For this review, take the finished solid that the model builds, in its own axes (mm). Face numbers are marked on the shaded views. Round coordinates to 2 decimals unless told otherwise and drop trailing zeros. Write each loop counter-clockwise with the first axis right and the second up, starting at its lowest first coordinate (ties: lowest second). Pieces come first, ordered by that corner, then holes. Notation, with made-up numbers: M -40,9.5 L -27,9.5 A13 cw -27,27.5 Z; hole C 45.5,79 d1. An arc over 180 degrees is marked long. Use one line per item in the form item = value. Start each with the question number.
Item 1: For P1, Ø1, axis at x = 5, y = 0.5, coming from the +Z side; P2, Ø2, axis at x = 25.5, y = 1, coming from the -Z side; P3, Ø3, axis at x = -30, z = 10, coming from the -Y side; P4, Ø0.6, axis at x = -25.5, y = 1, coming from the -Z side, all flat-tipped, find the tip position at first contact; note any pin that passes through.
Item 2: Draft analysis for pull direction X (two halves, no side actions). For the marked faces 1 and 2, state which applies: released by +X, released by -X, zero draft, split by the parting line, or undercut.
Item 3: Add section B-B (x = 30). Count the separate pieces of the cut face and the enclosed holes in it, and give its area (3 significant figures).
Item 4: For line 1 (X direction, y = 1.95, z = 10); line 2 (Z direction, x = 30, y = 1.8); line 3 (X direction, y = 1.7, z = 20), list the stretches that pass through material, from the lowest coordinate up. Write a range as [from, to].
Item 5: Add section A-A (y = 2.9). State the section outline as (x, z) points.
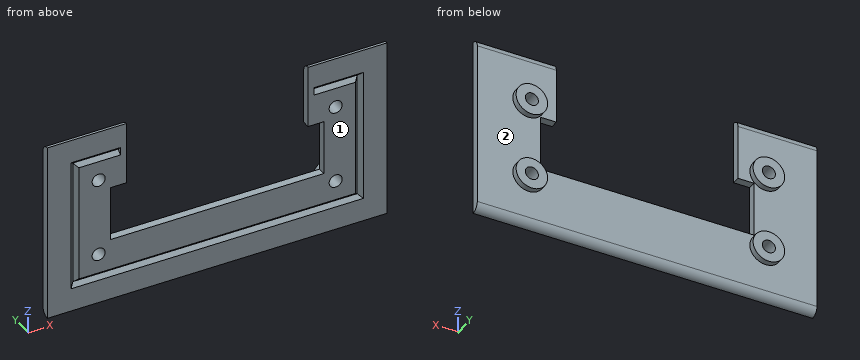
from build123d import *

# Parameters (mm, degrees)
SKETCH1_W               = 86
SKETCH1_H               = 46
BOSS_EXTRUDE1_DEPTH     = 2
SKETCH2_W               = 54
SKETCH2_H               = 14
CUT_EXTRUDE1_DEPTH      = 49.805737368
SKETCH4_R               = 4
BOSS_EXTRUDE2_DEPTH     = 1.5
CUT_EXTRUDE2_DEPTH      = 1.5
CUT_EXTRUDE2_DEPTH_BACK = 10
SKETCH3_R               = 1.65
SKETCH5_W               = 74
SKETCH5_H               = 34
SKETCH5_W_2             = 70
SKETCH5_H_2             = 30
CUT_EXTRUDE3_DEPTH      = 10
CUT_EXTRUDE3_TAPER      = 45
FILLET1_R               = 2
FILLET2_R               = 2
SKETCH6_W               = 46
SKETCH6_H               = 16
CUT_EXTRUDE4_DEPTH      = 10
BOSS_EXTRUDE3_START     = -1
SKETCH8_W               = 1.5
SKETCH8_H               = 2
BOSS_EXTRUDE3_DEPTH     = 1


with BuildPart() as part:
    # Sketch1 → Boss-Extrude1 (new body)
    with BuildSketch(Plane(origin=(0, 0, 0), x_dir=(1, 0, 0), z_dir=(0, 1, 0))):
        Rectangle(SKETCH1_W, SKETCH1_H)
    extrude(amount=BOSS_EXTRUDE1_DEPTH)

    # Sketch2 → Cut-Extrude1 (cut, through all)
    with BuildSketch(Plane(origin=(0, 2, 0), x_dir=(1, 0, 0), z_dir=(0, 1, 0))):
        Rectangle(SKETCH2_W, SKETCH2_H)
    extrude(amount=-CUT_EXTRUDE1_DEPTH, mode=Mode.SUBTRACT)

    # Sketch4 → Boss-Extrude2 (add)
    with BuildSketch(Plane(origin=(0, 2, 0), x_dir=(1, 0, 0), z_dir=(0, 1, 0))):
        with Locations(Location((-30, 10, 0), (0, 0, 270))):
            Circle(SKETCH4_R)
        with Locations(Location((-30, -10, 0), (0, 0, 90))):
            Circle(SKETCH4_R)
        with Locations(Location((30, -10, 0), (0, 0, 270))):
            Circle(SKETCH4_R)
        with Locations(Location((30, 10, 0), (0, 0, 90))):
            Circle(SKETCH4_R)
    extrude(amount=BOSS_EXTRUDE2_DEPTH)

    # Sketch3 → Cut-Extrude2 (cut, two sides: drawn at the far end of the back side and taken through both)
    with BuildSketch(Plane(origin=(0, 2, 0), x_dir=(1, 0, 0), z_dir=(0, 1, 0)).offset(-CUT_EXTRUDE2_DEPTH_BACK)):
        with Locations(Location((-30, 10, 0), (0, 0, 270))):
            Circle(SKETCH3_R)
        with Locations(Location((30, 10, 0), (0, 0, 270))):
            Circle(SKETCH3_R)
        with Locations(Location((30, -10, 0), (0, 0, 270))):
            Circle(SKETCH3_R)
        with Locations(Location((-30, -10, 0), (0, 0, 270))):
            Circle(SKETCH3_R)
    extrude(amount=CUT_EXTRUDE2_DEPTH + CUT_EXTRUDE2_DEPTH_BACK, mode=Mode.SUBTRACT)

    # Sketch5 → Cut-Extrude3 (cut)
    with BuildSketch(Plane.XZ):
        Rectangle(SKETCH5_W, SKETCH5_H)
        Rectangle(SKETCH5_W_2, SKETCH5_H_2, mode=Mode.SUBTRACT)
    extrude(amount=-CUT_EXTRUDE3_DEPTH, taper=CUT_EXTRUDE3_TAPER, mode=Mode.SUBTRACT)

    # Fillet1
    fillet1_edges = [part.edges().sort_by_distance(p)[0] for p in [
        (0, 2, -23),
    ]]
    fillet(fillet1_edges, radius=FILLET1_R - 0.0001)  # a hair under: the kernel refuses the full size

    # Fillet2
    fillet2_edges = [part.edges().sort_by_distance(p)[0] for p in [
        (0, 2, 23),
    ]]
    fillet(fillet2_edges, radius=FILLET2_R - 0.0001)  # a hair under: the kernel refuses the full size

    # Sketch6 → Cut-Extrude4 (cut)
    with BuildSketch(Plane(origin=(0, 2, 0), x_dir=(1, 0, 0), z_dir=(0, 1, 0))):
        with Locations((0, -15)):
            Rectangle(SKETCH6_W, SKETCH6_H)
    extrude(amount=-CUT_EXTRUDE4_DEPTH, mode=Mode.SUBTRACT)

    # Sketch8 → Boss-Extrude3 (add)
    with BuildSketch(Plane.XZ.offset(BOSS_EXTRUDE3_START)):
        with Locations((23.75, 16)):
            Rectangle(SKETCH8_W, SKETCH8_H)
        with Locations((-23.75, 16)):
            Rectangle(SKETCH8_W, SKETCH8_H)
    extrude(amount=BOSS_EXTRUDE3_DEPTH)


solid = part.part
Calculated:
q1.P1 = -7
q1.P2 = -23
q1.P3 = through
q1.P4 = -22.87
q2.face_1 = zero draft
q2.face_2 = undercut
q3.separate_pieces = 3
q3.enclosed_holes = 0
q3.area = 89.2 mm^2
q4.line_1 = [-43, -31.65], [-28.35, -23], [23, 28.35], [31.65, 43]
q4.line_2 = [-21.87, -11.65], [-8.35, 8.35], [11.65, 21.87]
q4.line_3 = [-43, -23], [23, 43]
q5.outline = C -30,-10 d8; C -30,10 d8; C 30,-10 d8; C 30,10 d8; hole C -30,-10 d3.3; hole C -30,10 d3.3; hole C 30,-10 d3.3; hole C 30,10 d3.3
